Source: CAD feature listing. Evaluate the final solid. Frame: model axes, mm. A direction names the side the tool comes from. Coordinates: 2 decimals unless noted, no trailing zeros. Order: outer loops, then holes, each group sorted by start corner. A loop starts at its lowest first (then second) coordinate and runs counter-clockwise, first axis right, second up. Notation, with made-up numbers: (60, 36) - (118, 36) arc R10 ccw to (118, 40) - close; hole circle Ø7 at (17.5, -37). An arc over 180 degrees is marked (long way). One line per question, with ' | ' between items.
from build123d import *

# Parameters (mm, degrees)
SKETCH7_R          = 2
CUT_EXTRUDE1_DEPTH = 10


with BuildPart() as part:
    # Sweep1: sweep along a path in Sketch4
    with BuildLine(Plane(origin=(0, 0, 0), x_dir=(0, 0, -1), z_dir=(1, 0, 0))) as sweep1_path:
        Line((0, 0), (220, 0))
        Line((220, 0), (220, 90))
    # Sketch2 → Sweep1 (sweep)
    with BuildSketch(Plane.XY):
        Polygon((0, 0), (30, 0), (30, 30), (27, 30), (27, 3), (0, 3), align=None)
    sweep(path=sweep1_path.line, transition=Transition.RIGHT)

    # Sketch7 → Cut-Extrude1 (cut)
    with BuildSketch(Plane(origin=(0, 0, -220), x_dir=(-1, 0, 0), z_dir=(0, 0, -1))):
        with Locations((-20, 85)):
            Circle(SKETCH7_R)
    extrude(amount=-CUT_EXTRUDE1_DEPTH, mode=Mode.SUBTRACT)


solid = part.part
(1) Set-up query: faces 1 (the flat face through (27, 28, -134)), 2 (the flat face through (15, 0, -112)). Return all of +Z, -Z, +X, -X, +Y, -Y with unobstructed straight access to the full face (end or side cutting, diameter ignored); none if empty.
Taken from the geometry:
face 1: +Z, -X, +Y | face 2: +Z, -Z, +X, -X, -Y
(2) Material intervals for L1, parallel to Y at x = 20, z = -217.85; L2, parallel to Z at x = 27.5, y = 50.5; L3, parallel to Z at x = 10, y = 67, sorted ascending. Write a range as from..to.
Taken from the geometry:
L1: y = 0..83, 87..90 | L2: z = -220..-190 | L3: z = -220..-217
(3) Pull-direction query (Y, two-part tool) for faces 3 (the cylindrical face through (20, 87, -219)), 4 (the flat face through (14, 3, -110)), 5 (the flat face through (0, 2, -111)); classes: pulls with the +Y half, pulls with the -Y half, needs draft (parallel to the pull), parting line crosses it, or undercut.
Taken from the geometry:
face 3: undercut | face 4: pulls with the +Y half | face 5: needs draft
(4) Cut plane B-B (x = 20). Return the cut outline in (y, z), and give its area (3 significant figures).
Taken from the geometry:
outline: (0, -220) - (83, -220) - (83, -217) - (3, -217) - (3, 0) - (0, 0) - close; (87, -220) - (90, -220) - (90, -217) - (87, -217) - close | area: 909 mm²
(5) Cut plane C-C (z = -196). Return the cut outline in (x, y).
Taken from the geometry:
outline: (0, 0) - (30, 0) - (30, 90) - (27, 90) - (27, 3) - (0, 3) - close
(6) Pin query (flat end, axial travel): P1, Ø0.9, axis at x = 28.5, z = -107, coming from the +Y side; P2, Ø1.5, axis at x = 11.5, z = -144.5, coming from the +Y side; P3, Ø1.5, axis at x = 28, y = 46, coming from the +Z side. Return the tip coordinate at first contact, or that it passes through.
Taken from the geometry:
P1: stops at y = 30 | P2: stops at y = 3 | P3: stops at z = -190
(7) Cut plane A-A (y = 85). Return the cut outline in (x, z), and give its area (3 significant figures).
Taken from the geometry:
outline: (0, -220) - (18, -220) - (18, -217) - (0, -217) - close; (22, -220) - (30, -220) - (30, -190) - (27, -190) - (27, -217) - (22, -217) - close | area: 159 mm²
(8) Cut plane D-D (x = 3). Return the cut outline in (y, z).
Taken from the geometry:
outline: (0, -220) - (90, -220) - (90, -217) - (3, -217) - (3, 0) - (0, 0) - close
